Autodesk Inventor part; units mm, degrees
ref_plane "YZ Plane" through (0, 0, 0) normal (1, 0, 0) x (0, 1, 0)
ref_plane "XZ Plane" through (0, 0, 0) normal (0, 1, 0) x (-1, 0, 0)
ref_plane "XY Plane" through (0, 0, 0) normal (0, 0, 1) x (1, 0, 0)
sketch "Sketch1" plane through (0, 0, 0) normal (0, 0, 1) x (1, 0, 0)
  line L0 (0, 0) -> (63.5, 0)
  line L1 (63.5, 0) -> (63.5, 19.05)
  line L2 (63.5, 19.05) -> (0, 19.05)
  line L3 (0, 19.05) -> (0, 0)
  dimension "d2" = 63.5
  dimension "d3" = 19.05
extrude "Stock Block" add sketch "Sketch1" along normal blind 41.275
sketch "Sketch2" plane through (0, 19.05, 0) normal (0, 1, 0) x (1, 0, 0)
  line L0 (63.5, 0) -> (0, 0)
  line L1 (0, 0) -> (0, -41.275)
  point P0 (31.75, -20.6375)
  dimension "d4" = 20.6375
  dimension "d5" = 31.75
hole "Mounting Hole" at (31.75, 19.05, 20.6375) direction (0, -1, 0) diameter 6.6548 end through all
sketch "Sketch3" plane through (0, 19.05, 0) normal (0, 1, 0) x (1, 0, 0)
  line L0 (6.35, -34.798) -> (6.35, -6.477) construction
  line L1 (3.048, -34.798) -> (3.048, -6.477)
  line L2 (9.652, -6.477) -> (9.652, -34.798)
  arc A0 (3.048, -34.798) -> (9.652, -34.798) centre (6.35, -34.798) ccw
  arc A1 (9.652, -6.477) -> (3.048, -6.477) centre (6.35, -6.477) ccw
  line L3 (0, 0) -> (0, -41.275)
  line L4 (63.5, -41.275) -> (0, -41.275)
  line L5 (63.5, 0) -> (0, 0)
  circle A2 centre (31.75, -20.6375) radius 3.3274
  line L6 (31.75, -20.6375) -> (31.75, 0) construction
  line L7 (57.15, -34.798) -> (57.15, -6.477) construction
  line L8 (60.452, -34.798) -> (60.452, -6.477)
  line L9 (53.848, -6.477) -> (53.848, -34.798)
  arc A3 (53.848, -34.798) -> (60.452, -34.798) centre (57.15, -34.798) ccw
  arc A4 (60.452, -6.477) -> (53.848, -6.477) centre (57.15, -6.477) ccw
  point P0 (6.35, -20.6375)
  point P1 (57.15, -20.6375)
  dimension "d13" = 6.604
  dimension "d15" = 3.175
  dimension "d16" = 3.175
  dimension "d24" = 25.4
extrude "Slots" cut sketch "Sketch3" against normal up to surface (19.05 mm away) contours L1 A1 L2 A0 | A3 L9 A4 L8
properties part number "Track Foot" material "Aluminum 6061"
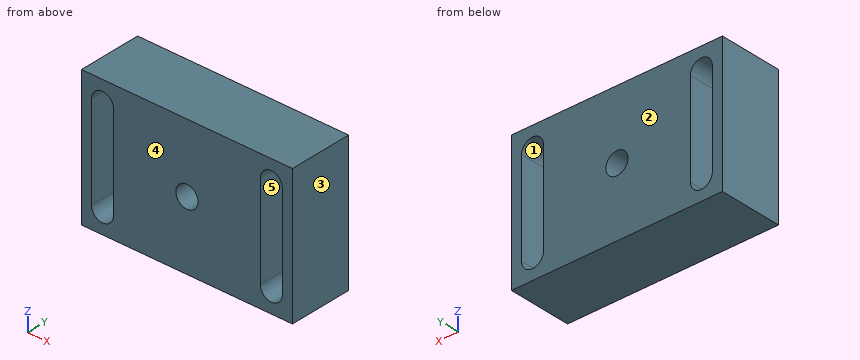
Could you check a few things on this model? Use its own coordinates, in mm. Face numbers are marked on the shaded views. A direction names the side the tool comes from. Round coordinates to 2 decimals unless told otherwise and drop trailing zeros. Order: outer loops, then holes, each group sorted by start corner. A loop starts at its lowest first (then second) coordinate and runs counter-clockwise, first axis right, second up. Notation, with made-up numbers: (77.25, 18) -> (86.25, 18) arc R18 ccw to (86.25, 53) -> close; hole circle Ø4 at (77.25, 87.25). An arc over 180 degrees is marked (long way). One line per question, with ' | ' between items.
Q1. If we section it at C-C on z = 14.5: Write out the boundary of the cut face in (x, y), plus the area to 3 significant figures.
Computed values:
outline: (0, 0) -> (3.05, 0) -> (3.05, 19.05) -> (0, 19.05) -> close; (9.65, 0) -> (53.85, 0) -> (53.85, 19.05) -> (9.65, 19.05) -> close; (60.45, 0) -> (63.5, 0) -> (63.5, 19.05) -> (60.45, 19.05) -> close | area: 958 mm²
Q2. If I drill on line 1 (X direction, y = 3, z = 30); line 2 (Z direction, x = 31.75, y = 7.75) (3 decimals); line 3 (X direction, y = 3, z = 20), over which ranges is the centre line in solid material (lowest first)? Write a range as from..to.
Computed values:
line 1: 0..3.05, 9.65..53.85, 60.45..63.5 | line 2: 0..17.31, 23.965..41.275 | line 3: 0..3.05, 9.65..28.48, 35.02..53.85, 60.45..63.5
Q3. If we section it at A-A on x = 6.35: Write out the boundary of the cut face in (y, z) (3 decimals), plus the area to 3 significant figures.
Computed values:
outline: (0, 0) -> (19.05, 0) -> (19.05, 3.175) -> (0, 3.175) -> close; (0, 38.1) -> (19.05, 38.1) -> (19.05, 41.275) -> (0, 41.275) -> close | area: 121 mm²
Q4. I'm going to push flat-ended pins straight in: pin 1 (5.5 mm diameter, centred on x = 31.75, z = 20.64, fed in from -Y); pin 2 (1.5 mm diameter, centred on x = 20.5, z = 4, fed in from -Y). Where does each tip first touch, or does it pass through?
Computed values:
pin 1: through | pin 2: y = 0
Q5. If we section it at D-D on x = 31.75: Write out the boundary of the cut face in (y, z) (3 decimals), plus the area to 3 significant figures.
Computed values:
outline: (0, 0) -> (19.05, 0) -> (19.05, 17.31) -> (0, 17.31) -> close; (0, 23.965) -> (19.05, 23.965) -> (19.05, 41.275) -> (0, 41.275) -> close | area: 660 mm²
Q6. We'd pull the mould along X, two halves only. Please class the marked faces 1, 2 and 3: released by +X, released by -X, zero draft, split by the parting line, or undercut.
Computed values:
face 1: undercut | face 2: zero draft | face 3: released by +X
Q7. Which directions (+Z, -Z, +X, -X, +Y, -Y) give clear straight access to the entire face, cutting with the end or side of a thin tool? Please do the marked faces 4 and 5.
Computed values:
face 4: +Z, -Z, +X, -X, -Y | face 5: +Y, -Y
Q8. If we section it at B-B on y = 16.5: Give the number of separate pieces and of enclosed holes in the cut face, plus the area to 3 significant figures.
Computed values:
separate pieces: 1 | enclosed holes: 3 | area: 2,140 mm²
